```python
from build123d import *

# Parameters (mm, degrees)
SKETCH_1_12_R       = 15
EXTRUDE_2_DEPTH     = 7
SKETCH_1_13_R       = 15
SKETCH_1_13_R_2     = 12.5
CUT_EXTRUDE_5_DEPTH = 4.9
M3X0_5_2_D          = 2.5


with BuildPart() as part:
    # ｽｹｯﾁ1<12> → ﾎﾞｽ - 押し出し2 (new body)
    with BuildSketch(Plane.XY):
        Circle(SKETCH_1_12_R)
        with BuildLine():
            Line((-2, 6.785786438), (-2, 5.656854249))
            ThreePointArc((-2, 5.656854249), (0, -6), (2, 5.656854249))
            Line((2, 5.656854249), (2, 6.785786438))
            ThreePointArc((2, 6.785786438), (2, 8.2), (0.585786438, 8.2))
            Line((0.585786438, 8.2), (-0.585786438, 8.2))
            ThreePointArc((-0.585786438, 8.2), (-2, 8.2), (-2, 6.785786438))
        make_face(mode=Mode.SUBTRACT)
    extrude(amount=-EXTRUDE_2_DEPTH)

    # ｽｹｯﾁ1<13> → ｶｯﾄ - 押し出し5 (cut)
    with BuildSketch(Plane.XY):
        Circle(SKETCH_1_13_R)
        Circle(SKETCH_1_13_R_2, mode=Mode.SUBTRACT)
    extrude(amount=-CUT_EXTRUDE_5_DEPTH, mode=Mode.SUBTRACT)

    # M3x0.5 ねじ穴2 (through all)
    with Locations(Plane(origin=(-6.540737726, 6.540737726, -7), x_dir=(-1, 0, 0), z_dir=(0, 0, -1))):
        with Locations((0, 0), (0, -13.081475452), (-13.081475452, -13.081475452), (-13.081475452, 0)):
            Hole(M3X0_5_2_D / 2)


solid = part.part
```
CAD build for the part. Positions are in the model's coordinates, mm. A direction names the side the tool comes from. Give positions to 0.01 mm unless a question says otherwise; leave off trailing zeros. Loops run counter-clockwise (first coordinate to the right, second up) from the corner with the lowest first, then second, coordinate; pieces in that order, holes last. Notation, with made-up numbers: M 15,35.25 L 69,35.25 A30 cw 69,71.25 Z; hole C -15,-15.5 d6. An arc over 180 degrees is marked long. Use one line per item in the form item = value.
Item 1: Drill centre lines: probe 1 along Y at (x, z) = (0.25, -0.25); probe 2 along Y at (x, z) = (5.5, -2.75); probe 3 along Y at (x, z) = (-6.25, -5). Where is each one in solid material? Low to high. Write a range as from..to.
Determined:
probe_1 = -12.5..-5.99, 8.2..12.5
probe_2 = -11.22..-7.23, -5.85..-2.4, 2.4..5.85, 7.23..11.22
probe_3 = -13.64..-7.76, -5.33..5.33, 7.76..13.64
Item 2: Slice it at C-C (z = -6.5). List the corners of the cut face in (x, y), plus the area to 3 significant figures.
Determined:
outline = C 0,0 d30; hole C -6.54,-6.54 d2.5; hole C -6.54,6.54 d2.5; hole M -2,5.66 A6 ccw long 2,5.66 L 2,6.79 A1 ccw 0.59,8.2 L -0.59,8.2 A1 ccw -2,6.79 Z; hole C 6.54,-6.54 d2.5; hole C 6.54,6.54 d2.5
area = 564 mm2
Item 3: Slice it at B-B (x = 0). List the corners of the cut face in (y, z).
Determined:
outline = M -15,-7 L -6,-7 L -6,0 L -12.5,0 L -12.5,-4.9 L -15,-4.9 Z; M 8.2,-7 L 15,-7 L 15,-4.9 L 12.5,-4.9 L 12.5,0 L 8.2,0 Z
Item 4: Which spindle directions (+Z, -Z, +X, -X, +Y, -Y) get a long thin tool onto all of the face, cutting with end or side? Do faces 1 (the face through (0, 8.2, -3)), 2 (the face through (5.4, 3, 0)), 3 (the face through (-3.4, 12.3, -4.9)). Say none if no direction does.
Determined:
face_1 = +Z, -Z
face_2 = +Z, +X, -X, +Y, -Y
face_3 = +Z
Item 5: Slice it at D-D (x = 6.75). List the corners of the cut face in (y, z).
Determined:
outline = M -13.4,-7 L -7.77,-7 L -7.77,0 L -10.52,0 L -10.52,-4.9 L -13.4,-4.9 Z; M -5.31,-7 L 5.31,-7 L 5.31,0 L -5.31,0 Z; M 7.77,-7 L 13.4,-7 L 13.4,-4.9 L 10.52,-4.9 L 10.52,0 L 7.77,0 Z
Item 6: Flat gauge pins, fed straight in: pin 1 (4 mm diameter, centred on x = -6.54, y = 6.54, fed in from -Z); pin 2 (2 mm diameter, centred on y = -5.5, z = -3.5, fed in from +X); pin 3 (2 mm diameter, centred on x = 6.54, y = 6.54, fed in from -Z); pin 4 (1.2 mm diameter, centred on y = 6.5, z = -2.5, fed in from -X). Where does each tip first touch, or does it go through?
Determined:
pin_1 = -7
pin_2 = 11.66
pin_3 = through
pin_4 = -11.02
Item 7: Slice it at A-A (y = 0). List the corners of the cut face in (x, z), plus the area to 4 significant figures.
Determined:
outline = M -15,-7 L -6,-7 L -6,0 L -12.5,0 L -12.5,-4.9 L -15,-4.9 Z; M 6,-7 L 15,-7 L 15,-4.9 L 12.5,-4.9 L 12.5,0 L 6,0 Z
area = 101.5 mm2
Item 8: Two-plate mould, pull along Y, no slides. Class faces 4 (the face through (11.923, 3.755, -2.416)), 5 (the face through (-6.7, 7.78, -3.45)), 6 (the face through (-0.2, -6.5, -7)): pulls with the +Y half, pulls with the -Y half, needs draft (parallel to the pull), parting line crosses it, or undercut.
Determined:
face_4 = parting line crosses it
face_5 = undercut
face_6 = needs draft
